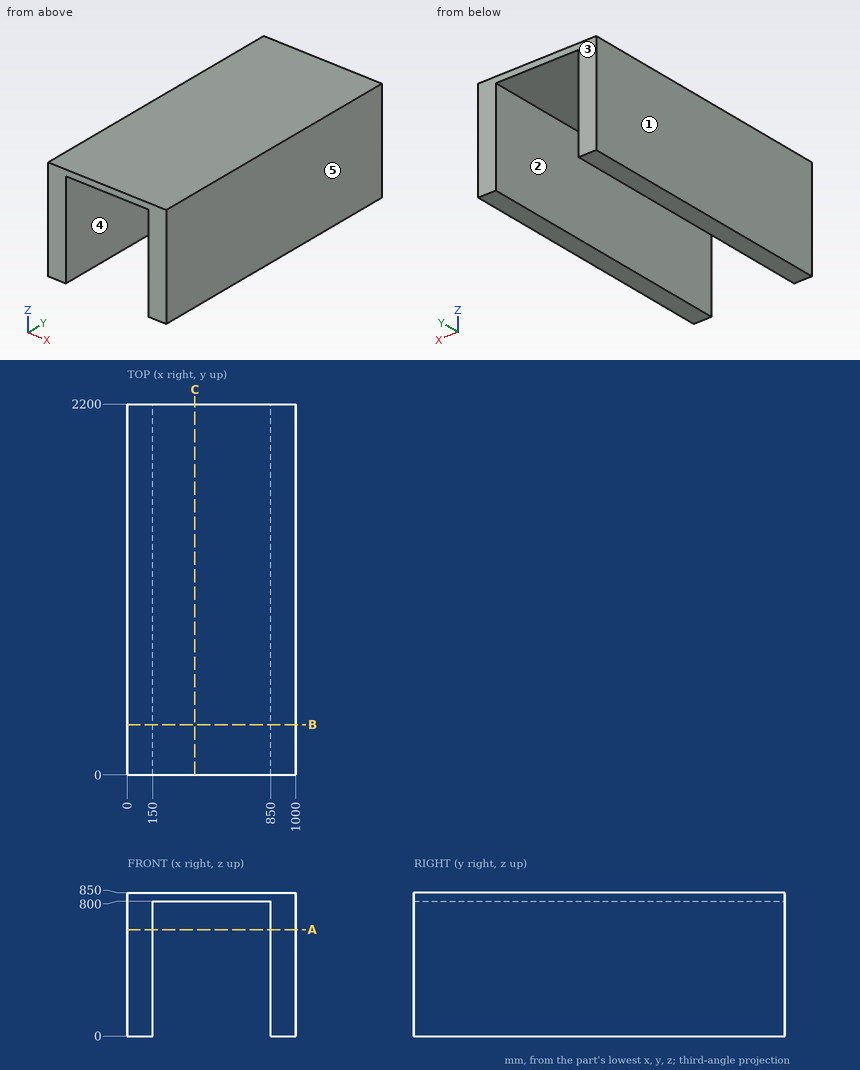
Could you check a few things on this drawing? It's one solid part, dimensions in mm from its lowest x, y, z. A direction names the side the tool comes from. Give positions to 0.01 mm unless a question says otherwise; leave off trailing zeros. Order: outer loops, then holes, each group sorted by start corner. A loop starts at its lowest first (then second) coordinate and runs counter-clockwise, first axis right, second up. Notation, with made-up numbers: (63, 17) -> (87, 17) arc R27 ccw to (87, 34) -> close; hole circle Ø3 at (86, -24.5). An arc over 180 degrees is marked (long way). Answer in a Markdown table with one row per item. Add a question column.
Item 1: Please list where these lines run through material, in increasing order: probe 1 along X at (y, z) = (473.5, 133); probe 2 along Z at (x, y) = (167, 1512).
Item 2: Imagine slicing it at B-B (y = 298). List the corners of the cut face in (x, z) for me.
Item 3: For the marked faces 4 and 5, which set-ups out of +Z, -Z, +X, -X, +Y, -Y let a thin tool reach every point of the face, with its end or its side?
Item 4: I'm going to push a flat-ended pin straight in: P1, Ø3, axis at x = 687, y = 491.5, coming from the -Z side. Where does the tip first touch, or does it pass through?
Item 5: We'd pull the mould along X, two halves only. Please class the marked faces 1, 2 and 3: pulls with the +X half, pulls with the -X half, needs draft (parallel to the pull), parting line crosses it, or undercut.
Item 6: Imagine slicing it at A-A (z = 631.5). List the corners of the cut face in (x, y) for me.
Item 7: Imagine slicing it at C-C (x = 400). List the corners of the cut face in (y, z) for me, and give its area (3 significant figures).
Result:
| question | item | result |
|---|---|---|
| 1 | probe 1 | 0 to 150, 850 to 1000 |
| 1 | probe 2 | 800 to 850 |
| 2 | outline | (0, 0) -> (150, 0) -> (150, 800) -> (850, 800) -> (850, 0) -> (1000, 0) -> (1000, 850) -> (0, 850) -> close |
| 3 | face 4 | -Z, +Y, -Y |
| 3 | face 5 | +Z, -Z, +X, +Y, -Y |
| 4 | P1 | z = 800 |
| 5 | face 1 | pulls with the -X half |
| 5 | face 2 | undercut |
| 5 | face 3 | needs draft |
| 6 | outline | (0, 0) -> (150, 0) -> (150, 2200) -> (0, 2200) -> close; (850, 0) -> (1000, 0) -> (1000, 2200) -> (850, 2200) -> close |
| 7 | outline | (0, 800) -> (2200, 800) -> (2200, 850) -> (0, 850) -> close |
| 7 | area | 110,000 mm2 |
